Part model, mm, in its own coordinate system. Face numbers are marked on the shaded views. A direction names the side the tool comes from. Give positions to 0.01 mm unless a question says otherwise; leave off trailing zeros. Loops run counter-clockwise (first coordinate to the right, second up) from the corner with the lowest first, then second, coordinate; pieces in that order, holes last. Notation, with made-up numbers: M 74,6.5 L 79,6.5 A23 cw 79,24.5 Z; hole C 29.25,-3.75 d9. An arc over 180 degrees is marked long. Put each result on its own line as item: value. Start each with the question number.
Autodesk Inventor part; units mm, degrees
ref_plane "YZ Plane" through (0, 0, 0) normal (1, 0, 0) x (0, 1, 0)
ref_plane "XZ Plane" through (0, 0, 0) normal (0, 1, 0) x (-1, 0, 0)
ref_plane "XY Plane" through (0, 0, 0) normal (0, 0, 1) x (1, 0, 0)
sketch "Sketch1" plane through (0, 0, 0) normal (0, 0, 1) x (1, 0, 0)
  line L0 (-13.5, 30.3) -> (-13.5, 55)
  line L1 (-13.5, 55) -> (-17.5, 55)
  line L2 (-17.5, 55) -> (-23.5, 49)
  line L3 (-23.5, 49) -> (-23.5, 0)
  line L4 (-23.5, 0) -> (-22.5, 0)
  line L5 (-22.5, 0) -> (-22.5, 2)
  line L6 (-22.5, 2) -> (-21.5, 2)
  line L7 (-21.5, 2) -> (-21.5, 4)
  line L8 (-21.5, 4) -> (-22.5, 4)
  line L9 (-22.5, 4) -> (-22.5, 30.3)
  line L10 (-22.5, 30.3) -> (-13.5, 30.3)
  line L11 (0, -11) -> (0, 66)
  point P0 (0, 0)
  point P1 (-23, 0)
  point P2 (-21.5, 3)
  dimension "d5" = 24.7
  dimension "d6" = 2
  dimension "d7" = 2
  dimension "d8" = 45
  dimension "d9" = 13.5
  dimension "d10" = 23.5
  dimension "d11" = 49
  dimension "d12" = 1
  dimension "d13" = 2
  dimension "d24" = 55
revolve "Revolution1" add sketch "Sketch1" angle 360 about axis through (0, -10, 0) along (0, 1, 0)
sketch "Sketch2" plane through (0, 55, 0) normal (0, 1, 0) x (1, 0, 0)
  line L0 (23.5, -23.5) -> (-2.5, -23.5)
  line L1 (-2.5, -23.5) -> (-2.5, 23.5)
  line L2 (-2.5, 23.5) -> (23.5, 23.5)
  line L3 (23.5, 23.5) -> (23.5, -23.5)
  circle A0 centre (0, 0) radius 23.5
  point P0 (-2.5, 0)
  point P1 (23.5, 0)
  point P2 (0, -23.5)
  point P3 (0, 23.5)
  point P4 (-2.5, 23.3666)
  point P5 (-2.5, -23.3666)
  dimension "d1" = 2.5
extrude "Extrusion1" cut sketch "Sketch2" against normal through all contours L0 A0 L3 | A0 L1 | A0 L2 L3 picked at (6.1667, 0)
sketch "Sketch3" plane through (0, 55, 0) normal (0, 1, 0) x (1, 0, 0)
  circle A0 centre (0, 0) radius 18.5 construction
  point P0 (-18.5, 0)
  point P1 (-9.25, 16.0215)
  point P2 (-9.25, -16.0215)
  dimension "d14" = 37
  dimension "d15" = 60
  dimension "d16" = 60
hole "Hole1" at (-18.5, 55, 0) at (-9.25, 55, -16.0215) at (-9.25, 55, 16.0215) direction (0, -1, 0) diameter 3.242 end through all counterbore diameter 7.2 counterbore depth 14.2
properties part number "Clamp" material "Brass, Soft Yellow, Welded"
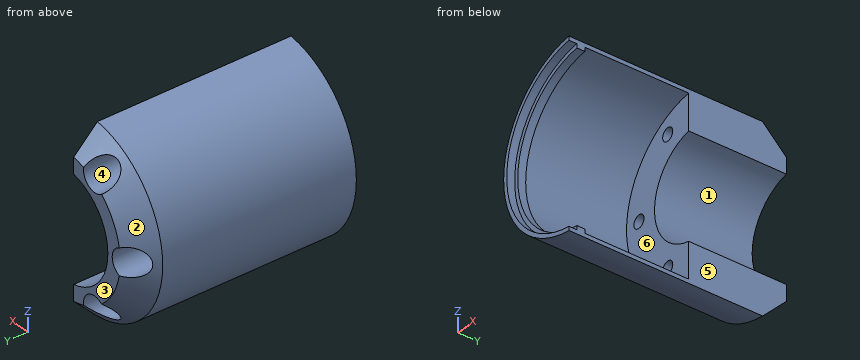
1) Band-saw the part on B-B on z = 0. Give the cut face in (x, y).
2) Band-saw the part on D-D on y = 46. Give the cut face in (x, z), then the cut area to 3 significant figures.
3) Band-saw the part on A-A on y = 31. Give the cut face in (x, z).
4) Pin check, flat tips, straight feed: pin 1 Ø2 at (x, z) = (-6.5, 17) entering from -Y; pin 2 Ø8 at (x, z) = (-10, 16) entering from +Y; pin 3 Ø5 at (y, z) = (19, 6.5) entering from +X; pin 4 Ø2 at (x, z) = (-17.5, 0) entering from +Y. Stop position of each tip, or through.
5) Mould opens along Z. For the marked faces 1, 2 and 3 say: +Z half, -Z half, draft (parallel to the pull), parting line (faces both ways), or undercut.
6) Band-saw the part on C-C on x = -9.25. State how many separate pieces and enclosed holes the cut face has, then the cut area to 3 significant figures.
7) Wall check: L1, parallel to Z at x = -9.25, y = 49.5; L2, parallel to Z at x = -9.25, y = 44.25; L3, parallel to X at y = 51, z = 15.5. Give the ranges that are in metal, low to high.
8) Which spindle directions (+Z, -Z, +X, -X, +Y, -Y) get a long thin tool onto all of the face, cutting with end or side? Do the marked faces 4, 5 and 6. Say none if no direction does.
Evaluation:
1. outline: M -23.5,0 L -22.5,0 L -22.5,2 L -21.5,2 L -21.5,4 L -22.5,4 L -22.5,30.3 L -20.12,30.3 L -20.12,40.8 L -22.1,40.8 L -22.1,50.4 L -23.5,49 Z; M -16.88,30.3 L -13.5,30.3 L -13.5,55 L -14.9,55 L -14.9,40.8 L -16.88,40.8 Z
2. outline: M -2.5,-23.37 L -2.5,-13.27 A13.5 cw -2.5,13.27 L -2.5,23.37 A23.5 ccw Z; hole C -18.5,0 d7.2; hole C -9.25,-16.02 d7.2; hole C -9.25,16.02 d7.2
2. area: 409 mm2
3. outline: M -2.5,-23.37 L -2.5,-13.27 A13.5 cw -2.5,13.27 L -2.5,23.37 A23.5 ccw Z; hole C -18.5,0 d3.24; hole C -9.25,-16.02 d3.24; hole C -9.25,16.02 d3.24
4. pin 1: y = 30.3
4. pin 2: y = 55
4. pin 3: x = -20.62
4. pin 4: y = 40.8
5. face 1: undercut
5. face 2: parting line
5. face 3: draft
6. separate pieces: 4
6. enclosed holes: 0
6. area: 359 mm2
7. L1: -21.06 to -19.62, -12.42 to -9.83, 9.83 to 12.42, 19.62 to 21.06
7. L2: -21.6 to -19.62, -12.42 to -9.83, 9.83 to 12.42, 19.62 to 21.6
7. L3: -14.9 to -12.81, -5.69 to -2.5
8. face 4: +Y
8. face 5: +Z, -Z, +X, +Y, -Y
8. face 6: +X
